Part model, mm, in its own coordinate system. A direction names the side the tool comes from. Give positions to 0.01 mm unless a question says otherwise; leave off trailing zeros. Order: outer loops, then holes, each group sorted by start corner. A loop starts at its lowest first (then second) coordinate and runs counter-clockwise, first axis right, second up. Notation, with made-up numbers: (15.25, 62) - (55.25, 62) arc R29 ccw to (55.25, 88) - close; hole circle Ø11 at (-5.5, 85.5). An arc over 180 degrees is marked (long way). One line per item, written item: value.
```python
from build123d import *

# Parameters (mm, degrees)
CROQUIS2_R            = 1.7
CORTAR_EXTRUIR1_DEPTH = 10
CROQUIS3_R            = 2.95
CORTAR_EXTRUIR2_DEPTH = 3
CROQUIS4_W            = 10
CROQUIS4_H            = 1
CORTAR_EXTRUIR3_DEPTH = 10


with BuildPart() as part:
    # Croquis1 → Revolución1 (revolve)
    with BuildSketch(Plane.XY):
        Polygon((21, 0), (21, 5), (29.2, 5), (29.2, 15), (30.2, 15), (30.2, 0), align=None)
    revolve(axis=Axis((0, 26.816952267, 0), (0, -1, 0)))

    # Croquis2 → Cortar-Extruir1 (cut)
    with BuildSketch(Plane(origin=(0, 5, 0), x_dir=(1, 0, 0), z_dir=(0, 1, 0))):
        with Locations((-24, 0)):
            Circle(CROQUIS2_R)
        with Locations((0, 24)):
            Circle(CROQUIS2_R)
        with Locations((24, 0)):
            Circle(CROQUIS2_R)
        with Locations((0, -24)):
            Circle(CROQUIS2_R)
    extrude(amount=-CORTAR_EXTRUIR1_DEPTH, mode=Mode.SUBTRACT)

    # Croquis3 → Cortar-Extruir2 (cut)
    with BuildSketch(Plane(origin=(0, 5, 0), x_dir=(1, 0, 0), z_dir=(0, 1, 0))):
        with Locations((-24, 0)):
            Circle(CROQUIS3_R)
        with Locations((0, 24)):
            Circle(CROQUIS3_R)
        with Locations((24, 0)):
            Circle(CROQUIS3_R)
        with Locations((0, -24)):
            Circle(CROQUIS3_R)
    extrude(amount=-CORTAR_EXTRUIR2_DEPTH, mode=Mode.SUBTRACT)

    # Croquis4 → Cortar-Extruir3 (cut)
    with BuildSketch(Plane(origin=(0, 15, 0), x_dir=(1, 0, 0), z_dir=(0, 1, 0))):
        with Locations((-29.2, 0)):
            Rectangle(CROQUIS4_W, CROQUIS4_H)
    extrude(amount=-CORTAR_EXTRUIR3_DEPTH, mode=Mode.SUBTRACT)


solid = part.part
```
1) Mould opens along X. For faces 1 (the cylindrical face through (-6.55, 7.4, -29.48)), 2 (the flat face through (26, 2, 0)), 3 (the flat face through (-21, 0, -6)) say: released by +X, released by -X, zero draft, split by the parting line, or undercut.
Outcome:
face 1: split by the parting line
face 2: undercut
face 3: zero draft
2) Cut at D-D, the plane y = 10.75. Give the cut face in (x, z).
Outcome:
outline: (-30.2, -0.5) arc R30.2 ccw (long way) to (-30.2, 0.5) - (-29.2, 0.5) arc R29.2 cw (long way) to (-29.2, -0.5) - close
3) Cut at A-A, the plane x = 0. Give the cut face in (y, z).
Outcome:
outline: (0, -30.2) - (15, -30.2) - (15, -29.2) - (5, -29.2) - (5, -26.95) - (2, -26.95) - (2, -25.7) - (0, -25.7) - close; (0, -22.3) - (2, -22.3) - (2, -21.05) - (5, -21.05) - (5, -21) - (0, -21) - close; (0, 21) - (5, 21) - (5, 21.05) - (2, 21.05) - (2, 22.3) - (0, 22.3) - close; (0, 25.7) - (2, 25.7) - (2, 26.95) - (5, 26.95) - (5, 29.2) - (15, 29.2) - (15, 30.2) - (0, 30.2) - close
4) Which spindle directions (+Z, -Z, +X, -X, +Y, -Y) get a long thin tool onto all of the face, cutting with end or side? Do faces 4 (the flat face through (0, 2, 26)), 5 (the cylindrical face through (-0.221, 1.014, 22.314)). Say none if no direction does.
Outcome:
face 4: +Y
face 5: +Y, -Y
5) Pin check, flat tips, straight feed: pin 1 (2 mm diameter, centred on x = 19, z = 13.5, fed in from +Y); pin 2 (1.5 mm diameter, centred on y = 12, z = 17, fed in from -X); pin 3 (4.5 mm diameter, centred on x = 24, z = 0, fed in from -Y); pin 4 (4 mm diameter, centred on x = 17.5, y = 13.5, fed in from -Z). Stop position of each tip, or through.
Outcome:
pin 1: stops at y = 5
pin 2: stops at x = -25.46
pin 3: stops at y = 0
pin 4: stops at z = -25.92
6) Drill centre lines: line 1 along Z through (x, y) = (0, 0.55); line 2 along Y through (x, z) = (-19, -22); line 3 along Z through (x, y) = (-17, 4). Where is each one in solid material? Low to high. Write a range as from..to.
Outcome:
line 1: z = -30.2..-25.7, -22.3..-21, 21..22.3, 25.7..30.2
line 2: y = 0..5
line 3: z = -24.96..-12.33, 12.33..24.96
7) Cut at B-B, the plane z = -6.5. Give the cut face in (x, y), then the cut area to 3 significant figures.
Outcome:
outline: (-29.49, 0) - (-19.97, 0) - (-19.97, 5) - (-28.47, 5) - (-28.47, 15) - (-29.49, 15) - close; (19.97, 0) - (29.49, 0) - (29.49, 15) - (28.47, 15) - (28.47, 5) - (19.97, 5) - close
area: 116 mm^2
8) Cut at C-C, the plane x = 14.5. Give the cut face in (y, z), then the cut area to 3 significant figures.
Outcome:
outline: (0, -26.49) - (15, -26.49) - (15, -25.35) - (5, -25.35) - (5, -15.19) - (0, -15.19) - close; (0, 15.19) - (5, 15.19) - (5, 25.35) - (15, 25.35) - (15, 26.49) - (0, 26.49) - close
area: 136 mm^2
